The figure shows three views and two pictorial views of one solid part (mm, origin at its lowest corner). Answer the questions. Give positions to 0.01 mm unless a question says otherwise; leave off trailing zeros. Loops run counter-clockwise (first coordinate to the right, second up) from the corner with the lowest first, then second, coordinate; pieces in that order, holes last. Notation, with made-up numbers: M 49.5,19 L 78.5,19 A9 ccw 78.5,36 Z; hole C 82.25,-9 d10. An arc over 180 degrees is marked long. Write item = value, one per line. Start each with the question number.
1. Section B-B on y = 10.25 is taken. Determine the outline of the cut face in (x, z), plus the area to 3 significant figures.
2. Section A-A on x = 0.3 is taken. Determine the outline of the cut face in (y, z), plus the area to 4 significant figures.
3. Consider L1, parallel to Z at x = 0.15, y = 13; L2, parallel to Y at x = 0.35, z = 0.65. Determine where each line is inside the solid, lowest interval first. Write a range as [from, to].
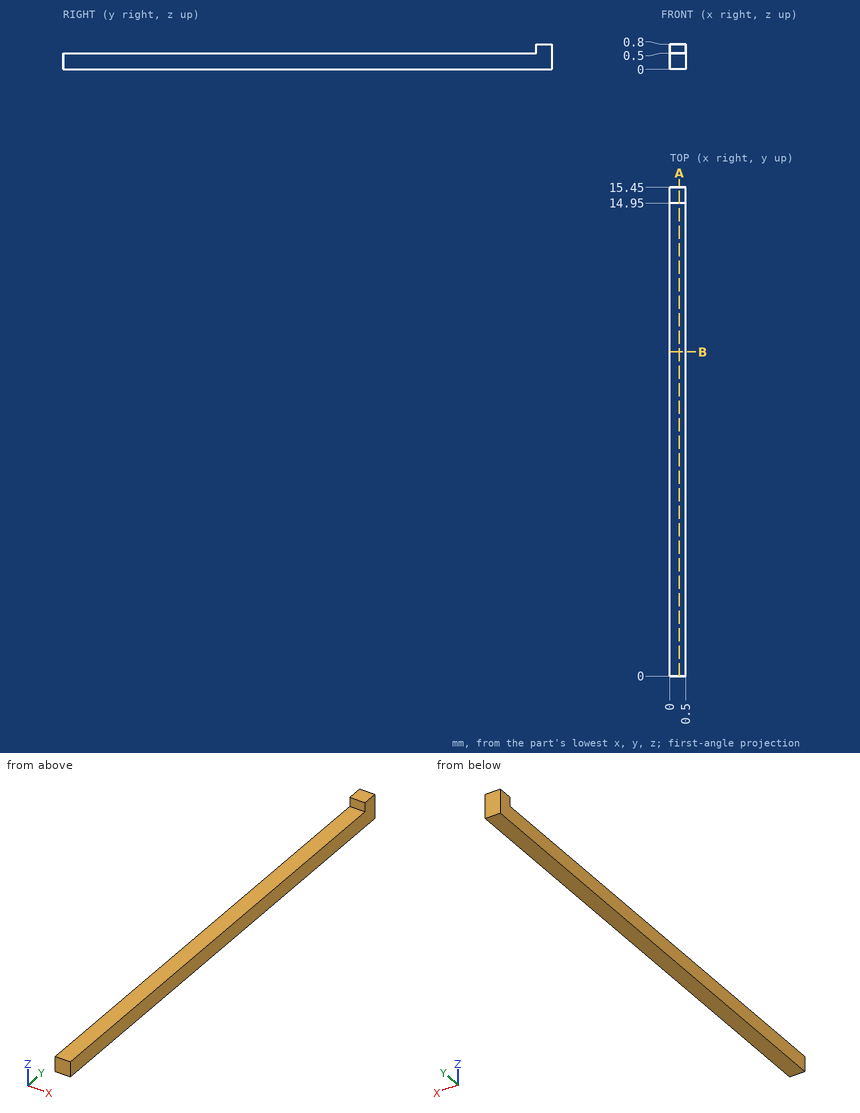
Verdict:
q1.outline = M 0,0 L 0.5,0 L 0.5,0.5 L 0,0.5 Z
q1.area = 0.250 mm2
q2.outline = M 0,0 L 15.45,0 L 15.45,0.8 L 14.95,0.8 L 14.95,0.5 L 0,0.5 Z
q2.area = 7.875 mm2
q3.L1 = [0, 0.5]
q3.L2 = [14.95, 15.45]
